Read the model definition and answer for the solid it produces. Units are mm, in the model's axes. Face numbers are marked on the shaded views. A direction names the side the tool comes from. Round coordinates to 2 decimals unless told otherwise and drop trailing zeros. Loops run counter-clockwise (first coordinate to the right, second up) from the corner with the lowest first, then second, coordinate; pieces in that order, holes last. Notation, with made-up numbers: (4, 33.25) - (29, 33.25) arc R21 cw to (29, 50.25) - close; hole circle Ø5 at (-5, -18.75). An arc over 180 degrees is marked (long way). Use CSV: the item, a comma, the result in double quotes. Start each with the question number.
1. Consider line 1 along Z through (x, y) = (-52.5, 10.75); line 2 along X through (y, z) = (-8, 35); line 3 along X through (y, z) = (-8.85, 25). Determine where each line is inside the solid, lowest interval first.
2. Find section A-A (x = -52.5). Give the vertices of the cut face in (y, z).
3. Find section D-D (x = 63). Give the vertices of the cut face in (y, z).
4. Find section B-B (z = 15). Give the vertices of the cut face in (x, y).
5. Find section C-C (y = 0). Give the vertices of the cut face in (x, z).
6. Given pin 1 Ø8 at (y, z) = (1.5, -2.5) entering from -X; pin 2 Ø1 at (y, z) = (2, -10) entering from -X; pin 3 Ø8 at (x, z) = (-52.5, 15) entering from -Y; pin 4 Ø8 at (y, z) = (7, -16) entering from +X, each flat-ended and moving along its own axis, determine where each tip first touches the part or whether it passes through.
7. A tool of negligible diameter and unlimited length cuts with its end or side. For the marked faces 1 and 2, from which of +Z, -Z, +X, -X, +Y, -Y can it reach the whole face along a straight path? Write none if from no direction.
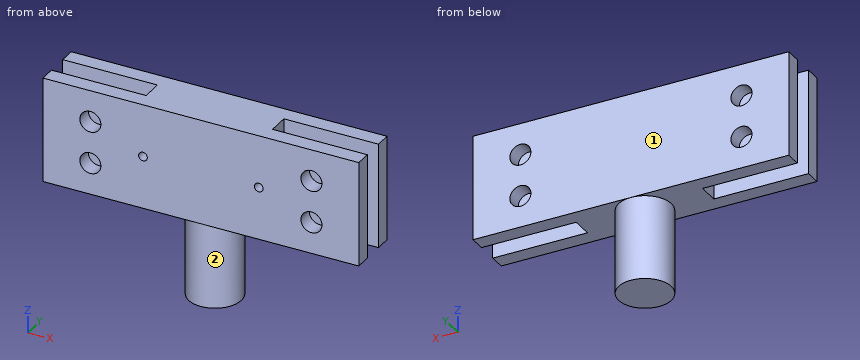
Autodesk Inventor part; units mm, degrees
ref_plane "YZ Plane" through (0, 0, 0) normal (1, 0, 0) x (0, 1, 0)
ref_plane "XZ Plane" through (0, 0, 0) normal (0, 1, 0) x (-1, 0, 0)
ref_plane "XY Plane" through (0, 0, 0) normal (0, 0, 1) x (1, 0, 0)
sketch "Esboço1" plane through (0, 0, 0) normal (0, 0, 1) x (1, 0, 0)
  circle A0 centre (0, 0) radius 12.5
  arc A1 (0, 12.5) -> (0, 12.5) centre (0, 0) ccw
  line L0 (0, 12.5) -> (75, 12.5)
  line L1 (75, 12.5) -> (75, 5)
  line L2 (0, -12.5) -> (75, -12.5)
  line L3 (75, -12.5) -> (75, -5)
  line L4 (75, 5) -> (30, 5)
  line L5 (30, -5) -> (75, -5)
  line L6 (75, -5) -> (75, 5) construction
  line L7 (75, 0) -> (28.253, 0) construction
  line L8 (0, 0) -> (-5.8343, 0) construction
  arc A2 (11.9242, 3.75) -> (0, 12.5) centre (0, 0) ccw construction
  arc A3 (0, -12.5) -> (11.9242, -3.75) centre (0, 0) ccw construction
  arc A4 (11.9242, -3.75) -> (11.9242, 3.75) centre (0, 0) ccw construction
  line L9 (0, 0) -> (0, 31.0423) construction
  line L10 (0, 12.5) -> (-75, 12.5)
  line L11 (0, -12.5) -> (-75, -12.5)
  line L12 (-75, -12.5) -> (-75, -5)
  line L13 (-75, 5) -> (-30, 5)
  line L14 (-30, -5) -> (-75, -5)
  line L15 (-75, 5) -> (-75, 12.5)
  arc A5 (0, 12.5) -> (-11.9242, 3.75) centre (0, 0) ccw construction
  arc A6 (-11.9242, 3.75) -> (-11.9242, -3.75) centre (0, 0) ccw construction
  arc A7 (-11.9242, -3.75) -> (0, -12.5) centre (0, 0) ccw construction
  arc A8 (0, -12.5) -> (0, -12.5) centre (0, 0) ccw
  line L16 (30, -5) -> (30, 5)
  line L17 (-30, -5) -> (-30, 5)
  arc A9 (0, 12.5) -> (0, 12.5) centre (0, 22.5) ccw
  arc A10 (0, -12.5) -> (0, -12.5) centre (0, -22.5) ccw
  arc A11 (0, -12.5) -> (0, -12.5) centre (0, -22.5) ccw
  arc A12 (0, 12.5) -> (0, 12.5) centre (0, 22.5) ccw
  line L18 (-30, 0) -> (30, 0)
  line L19 (0, 0) -> (0, 17) construction
  dimension "d0" = 25
  dimension "d1" = 25
  dimension "d6" = 10
  dimension "d7" = 7.5
  dimension "d8" = 7.5
  dimension "d10" = 10
  dimension "d13" = 150
  dimension "d45" = 60
extrude "Extrusão1" add sketch "Esboço1" along normal blind 50 contours L18 A0 | L18 L16 L5 L3 L2 A0 | A0 L0 L1 L4 L16 L18 | A0 L18 | A0 L18 L17 L13 L15 L10 | L11 L12 L14 L17 L18 A0
extrude "Extrusão2" add sketch "Esboço1" against normal blind 40 contours L18 A0 | A0 L18
sketch "Esboço2" plane through (0, 12.5, 0) normal (0, 1, 0) x (1, 0, 0)
  circle A0 centre (52.5, -15) radius 5
  circle A1 centre (-52.5, -15) radius 5
  line L0 (75, 0) -> (75, -50)
  line L1 (-75, 0) -> (-75, -50)
  circle A2 centre (-52.5, -35) radius 5
  circle A3 centre (52.5, -35) radius 5
  line L2 (0, 0) -> (-75, 0)
  line L3 (-52.5, -35) -> (-52.5, -15) construction
  line L4 (75, 0) -> (0, 0)
  line L5 (52.5, -35) -> (52.5, -15) construction
  dimension "d17" = 10
  dimension "d18" = 10
  dimension "d22" = 150
  dimension "d23" = 22.5
  dimension "d29" = 22.5
  dimension "d38" = 10
  dimension "d40" = 20
  dimension "d41" = 10
  dimension "d44" = 20
  dimension "d63" = 15
  dimension "d64" = 15
extrude "Extrusão3" cut sketch "Esboço2" against normal up to surface (25 mm away)
sketch "Esboço4" plane through (-75, -12.5, 50) normal (0, -1, 0) x (1, 0, 0)
  circle A0 centre (47.5, -25) radius 2.5
  circle A1 centre (102.5, -25) radius 2.5
  line L0 (47.5, -25) -> (102.5, -25)
  line L1 (75, -25) -> (75, -15.8254)
  line L2 (150, 0) -> (0, 0)
  line L3 (75, 0) -> (75, 11.0535)
  line L4 (0, -50) -> (0, 0)
  line L5 (0, -25) -> (-11.4925, -25)
  point P0 (75, -50)
  dimension "d53" = 5
  dimension "d54" = 5
  dimension "d55" = 55
hole "Furo2" at (-27.5, -12.5, 25) at (27.5, -12.5, 25) direction (0, 1, 0) diameter 4.134 depth 5 tip angle 118
equation "\"d8\" = d7"
equation "\"d29\" = d23"
equation "\"d38\" = d18"
equation "\"d41\" = d17"
properties part number "Junta"
Filled sheet:
1,line 1,"z = 0 to 10, 20 to 30, 40 to 50"
1,line 2,"x = -75 to -57.5, -47.5 to 47.5, 57.5 to 75"
1,line 3,"x = -75 to -29.57, -25.43 to 25.43, 29.57 to 75"
2,outline,"(-12.5, 0) - (-5, 0) - (-5, 10) - (-12.5, 10) - close; (-12.5, 20) - (-5, 20) - (-5, 30) - (-12.5, 30) - close; (-12.5, 40) - (-5, 40) - (-5, 50) - (-12.5, 50) - close; (5, 0) - (12.5, 0) - (12.5, 10) - (5, 10) - close; (5, 20) - (12.5, 20) - (12.5, 30) - (5, 30) - close; (5, 40) - (12.5, 40) - (12.5, 50) - (5, 50) - close"
3,outline,"(-12.5, 0) - (-5, 0) - (-5, 50) - (-12.5, 50) - close; (5, 0) - (12.5, 0) - (12.5, 50) - (5, 50) - close"
4,outline,"(-75, -12.5) - (-57.5, -12.5) - (-57.5, -5) - (-75, -5) - close; (-75, 5) - (-57.5, 5) - (-57.5, 12.5) - (-75, 12.5) - close; (-47.5, -12.5) - (47.5, -12.5) - (47.5, -5) - (30, -5) - (30, 5) - (47.5, 5) - (47.5, 12.5) - (-47.5, 12.5) - (-47.5, 5) - (-30, 5) - (-30, -5) - (-47.5, -5) - close; (57.5, -12.5) - (75, -12.5) - (75, -5) - (57.5, -5) - close; (57.5, 5) - (75, 5) - (75, 12.5) - (57.5, 12.5) - close"
5,outline,"(-30, 0) - (-12.5, 0) - (-12.5, -40) - (12.5, -40) - (12.5, 0) - (30, 0) - (30, 50) - (-30, 50) - close"
6,pin 1,"stops at x = -30"
6,pin 2,"stops at x = -12.41"
6,pin 3,"passes through"
6,pin 4,"stops at x = 12.13"
7,face 1,"+Z, -Z, +X, -X, +Y"
7,face 2,"-Z"
